Part model, mm, in its own coordinate system. Face numbers are marked on the shaded views. A direction names the side the tool comes from. Coordinates: 2 decimals unless noted, no trailing zeros. Write each loop counter-clockwise with the first axis right and the second up, starting at its lowest first coordinate (ties: lowest second). Pieces come first, ordered by that corner, then holes. Notation, with made-up numbers: M 69.5,-15.5 L 98.5,-15.5 A20 ccw 98.5,8.5 Z; hole C 53,40 d10. An arc over 180 degrees is marked long. Use a Markdown table: item, result. Add a question column.
Q1. Wall check: L1, parallel to Z at x = 0, y = 1.35; L2, parallel to Y at x = 0, z = -6.75; L3, parallel to Y at x = 6, z = -12. Give the ranges that are in metal, low to high. Write a range as from..to.
Q2. Slice it at B-B on y = -29. Write the cut outline in (x, z).
Q3. Tool access for the marked faces 1, 2, 3 and 4: list every direction of +Z, -Z, +X, -X, +Y, -Y with a clear straight run to the whole face (end or side of a thin tool).
Q4. Pin check, flat tips, straight feed: pin 1 Ø2.5 at (x, y) = (2, 18.5) entering from -Z; pin 2 Ø5 at (x, y) = (0, 50) entering from -Z; pin 3 Ø8 at (x, y) = (2.5, 32.5) entering from +Z. Stop position of each tip, or through.
Q5. Slice it at C-C on y = 7. Write the cut outline in (x, z), then the cut area to 3 significant figures.
Q6. Slice it at A-A on y = 50. Count the separate pieces of the cut face and the enclosed holes in it, then the cut area to 3 significant figures.
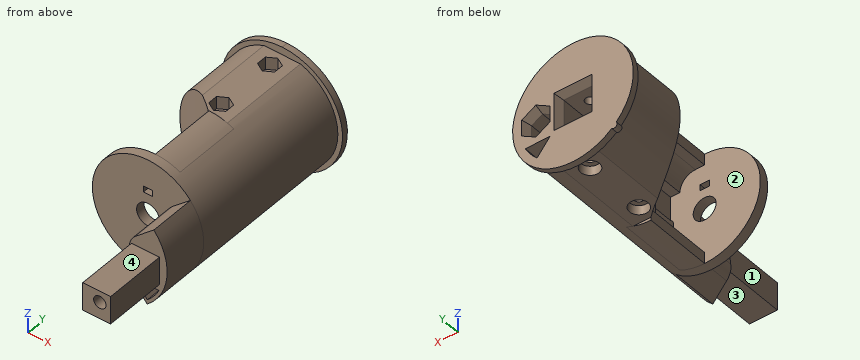
from build123d import *
from build123d.topology import SkipClean

# Parameters (mm, degrees)
SKETCH_1_R          = 18
EXTRUDE_1_DEPTH     = 55
SKETCH_2_R          = 19.5
EXTRUDE_2_DEPTH     = 2
SKETCH_3_W          = 10.25
SKETCH_3_H          = 10.25
CUT_EXTRUDE_1_DEPTH = 40
EXTRUDE_START       = 15
EXTRUDE_3_DEPTH     = 15
BOSS_EXTRUDE1_START = 20
SKETCH1_R           = 18
BOSS_EXTRUDE1_DEPTH = 20
BOSS_EXTRUDE2_START = 7
SKETCH3_R           = 18
BOSS_EXTRUDE2_DEPTH = 7
SKETCH4_W           = 10.2
SKETCH4_H           = 10.2
CUT_EXTRUDE2_DEPTH  = 27
CUT_EXTRUDE4_DEPTH  = 25
BOSS_EXTRUDE3_DEPTH = 3
SKETCH9_W           = 36
SKETCH9_H           = 22
CUT_EXTRUDE5_DEPTH  = 8
SKETCH10_R          = 3.7
SKETCH10_W          = 3
SKETCH10_H          = 2
CUT_EXTRUDE6_DEPTH  = 10
SKETCH11_R          = 2
CUT_EXTRUDE7_DEPTH  = 102
SKETCH15_R          = 18
CUT_EXTRUDE9_DEPTH  = 27
CUT_EXTRUDE11_DEPTH = 30
SKETCH18_R          = 1.5
CUT_EXTRUDE12_DEPTH = 71.437915926
SKETCH19_R          = 3
CUT_EXTRUDE13_DEPTH = 3
BOSS_EXTRUDE5_DEPTH = 22
CUT_EXTRUDE16_DEPTH = 4
CUT_EXTRUDE17_DEPTH = 25.4
CUT_EXTRUDE18_DEPTH = 71.437915926
FILLET2_R           = 5
SKETCH30_W          = 18.8
SKETCH30_H          = 10
CUT_EXTRUDE20_DEPTH = 3
CHAMFER1_SIZE       = 1
CHAMFER1_SIZE2      = 2.747477419
CHAMFER2_SIZE       = 1
CHAMFER2_SIZE2      = 2.747477419
BOSS_EXTRUDE7_START = 20
SKETCH37_W          = 9
SKETCH37_H          = 9
SKETCH37_R          = 2
BOSS_EXTRUDE7_DEPTH = 20
CUT_EXTRUDE22_DEPTH = 15
CUT_EXTRUDE23_DEPTH = 78.100583655
SKETCH40_W          = 4.363156696
SKETCH40_H          = 4.363156696
CUT_EXTRUDE24_DEPTH = 10
FILLET7_R           = 6
BOSS_EXTRUDE8_DEPTH = 2
CUT_EXTRUDE25_DEPTH = 12


with BuildPart() as part:
    # Эскиз1 → Бобышка-Вытянуть1 (new body)
    with BuildSketch(Plane(origin=(0, 0, 0), x_dir=(1, 0, 0), z_dir=(0, 1, 0))):
        with Locations(Location((0, 0, 0), (0, 0, 270))):
            Circle(SKETCH_1_R)
    extrude(amount=EXTRUDE_1_DEPTH)

    # Эскиз2 → Бобышка-Вытянуть2 (add)
    with BuildSketch(Plane(origin=(0, 55, 0), x_dir=(1, 0, 0), z_dir=(0, 1, 0))):
        with Locations(Location((0, 0, 0), (0, 0, 270))):
            Circle(SKETCH_2_R)
    extrude(amount=EXTRUDE_2_DEPTH)

    # Эскиз3 → Вырез-Вытянуть1 (cut)
    with BuildSketch(Plane(origin=(0, 57, 0), x_dir=(1, 0, 0), z_dir=(0, 1, 0))):
        Rectangle(SKETCH_3_W, SKETCH_3_H)
    extrude(amount=-CUT_EXTRUDE_1_DEPTH, mode=Mode.SUBTRACT)

    # Эскиз4 → Бобышка-Вытянуть3 (add)
    with SkipClean():  # the faces are left unmerged after this step: merging them gives an invalid solid
        with BuildSketch(Plane.XZ.offset(EXTRUDE_START)):
            with BuildLine():
                Line((5.142300877, -6.128355545), (11.570176974, -13.788799976))
                ThreePointArc((11.570176974, -13.788799976), (17.937391115, -1.5), (13.69961987, 11.675633406))
                Line((13.69961987, 11.675633406), (5.142300877, 4.38257561))
                Line((5.142300877, 4.38257561), (5.142300877, -6.128355545))
            make_face()
        extrude(amount=-EXTRUDE_3_DEPTH)

    # Sketch1 → Boss-Extrude1 (add)
    with BuildSketch(Plane.XZ.offset(15).offset(BOSS_EXTRUDE1_START)):
        with Locations(Location((0, 0, 0), (0, 0, 270))):
            Circle(SKETCH1_R)
    extrude(amount=-BOSS_EXTRUDE1_DEPTH)

    # Sketch3 → Boss-Extrude2 (add)
    with BuildSketch(Plane.XZ.offset(35).offset(BOSS_EXTRUDE2_START)):
        with Locations(Location((0, 0, 0), (0, 0, 270))):
            Circle(SKETCH3_R)
    extrude(amount=-BOSS_EXTRUDE2_DEPTH)

    # Sketch4 → Cut-Extrude2 (cut)
    with BuildSketch(Plane.XZ.offset(42)):
        Rectangle(SKETCH4_W, SKETCH4_H)
    extrude(amount=-CUT_EXTRUDE2_DEPTH, mode=Mode.SUBTRACT)

    # Sketch6 → Cut-Extrude4 (cut)
    with BuildSketch(Plane.XZ):
        with BuildLine():
            Line((0, 18), (0, -18))
            ThreePointArc((0, -18), (-18, 0), (0, 18))
        make_face()
    extrude(amount=-CUT_EXTRUDE4_DEPTH, mode=Mode.SUBTRACT)

    # Sketch8 → Boss-Extrude3 (add)
    with BuildSketch(Plane.XZ):
        with BuildLine():
            Line((0, -18), (0, 18))
            ThreePointArc((0, 18), (-18, 0), (0, -18))
        make_face()
    extrude(amount=-BOSS_EXTRUDE3_DEPTH)

    # Sketch9 → Cut-Extrude5 (cut)
    with BuildSketch(Plane.ZY):
        with Locations((0, 14)):
            Rectangle(SKETCH9_W, SKETCH9_H)
    extrude(amount=-CUT_EXTRUDE5_DEPTH, mode=Mode.SUBTRACT)

    # Sketch10 → Cut-Extrude6 (cut)
    with BuildSketch(Plane.XZ):
        with Locations(Location((0, 0, 0), (0, 0, 270))):
            Circle(SKETCH10_R)
        with Locations((0, 7.7)):
            Rectangle(SKETCH10_W, SKETCH10_H)
    extrude(amount=-CUT_EXTRUDE6_DEPTH, mode=Mode.SUBTRACT)

    # Sketch11 → Cut-Extrude7 (cut)
    with BuildSketch(Plane.XZ.offset(42)):
        with Locations(Location((12, 0, 0), (0, 0, 270))):
            Circle(SKETCH11_R)
    extrude(amount=-CUT_EXTRUDE7_DEPTH, mode=Mode.SUBTRACT)

    # Sketch15 → Cut-Extrude9 (cut)
    with BuildSketch(Plane.XZ.offset(42)):
        with Locations(Location((0, 0, 0), (0, 0, 310))):
            Circle(SKETCH15_R)
    extrude(amount=-CUT_EXTRUDE9_DEPTH, mode=Mode.SUBTRACT)

    # Sketch17 → Cut-Extrude11 (cut)
    with BuildSketch(Plane.XZ.offset(-25)):
        with BuildLine():
            Line((5.916079783, -17), (-5.916079783, -17))
            ThreePointArc((-5.916079783, -17), (0, -18), (5.916079783, -17))
        make_face()
        with BuildLine():
            Line((5.916079783, 17), (-5.916079783, 17))
            ThreePointArc((-5.916079783, 17), (0, 18), (5.916079783, 17))
        make_face()
    extrude(amount=-CUT_EXTRUDE11_DEPTH, mode=Mode.SUBTRACT)

    # Sketch18 → Cut-Extrude12 (cut, through all)
    with BuildSketch(Plane.XY.offset(-17)):
        with Locations(Location((0, 30, 0), (0, 0, 180))):
            Circle(SKETCH18_R)
        with Locations(Location((0, 50, 0), (0, 0, 180))):
            Circle(SKETCH18_R)
    extrude(amount=CUT_EXTRUDE12_DEPTH, mode=Mode.SUBTRACT)

    # Sketch19 → Cut-Extrude13 (cut)
    with BuildSketch(Plane.XY.offset(-17)):
        with Locations((0, 30)):
            Circle(SKETCH19_R)
        with Locations((0, 50)):
            Circle(SKETCH19_R)
    extrude(amount=CUT_EXTRUDE13_DEPTH, mode=Mode.SUBTRACT)

    # Sketch23 → Boss-Extrude5 (add)
    with BuildSketch(Plane(origin=(0, 3, 0), x_dir=(1, 0, 0), z_dir=(0, 1, 0))):
        with BuildLine():
            Line((0, -14.4), (8, -14.4))
            Line((8, -14.4), (8, -16.124515497))
            ThreePointArc((8, -16.124515497), (4.108449894, -17.524857759), (0, -18))
            Line((0, -18), (0, -14.4))
        make_face()
        with BuildLine():
            Line((0, 14.4), (8, 14.4))
            Line((8, 14.4), (8, 16.124515497))
            ThreePointArc((8, 16.124515497), (4.108449894, 17.524857759), (0, 18))
            Line((0, 18), (0, 14.4))
        make_face()
    extrude(amount=BOSS_EXTRUDE5_DEPTH)

    # Sketch25 → Cut-Extrude16 (cut)
    with BuildSketch(Plane.XY.offset(17)):
        Polygon((2.771281292, 28.4), (2.771281292, 31.6), (0, 33.2), (-2.771281292, 31.6), (-2.771281292, 28.4), (0, 26.8), align=None)
        Polygon((-2.782126929, 48.418933983), (-0.021820128, 46.800074394), (2.760306801, 48.381140412), (2.782126929, 51.581066017), (0.021820128, 53.199925606), (-2.760306801, 51.618859588), align=None)
    extrude(amount=-CUT_EXTRUDE16_DEPTH, mode=Mode.SUBTRACT)

    # Sketch26 → Cut-Extrude17 (cut)
    with BuildSketch(Plane(origin=(0, 57, 0), x_dir=(1, 0, 0), z_dir=(0, 1, 0))):
        Polygon((8.449295844, -2.05), (12, -4.1), (15.550704156, -2.05), (15.550704156, 2.05), (12, 4.1), (8.449295844, 2.05), align=None)
    extrude(amount=-CUT_EXTRUDE17_DEPTH, mode=Mode.SUBTRACT)

    # Sketch27 → Cut-Extrude18 (cut, through all)
    with BuildSketch(Plane.XY.offset(17)):
        with BuildLine():
            Line((-20, 36.547005384), (-20, 25))
            Line((-20, 25), (0, 25))
            ThreePointArc((0, 25), (-9.324199199, 31.944024015), (-20, 36.547005384))
        make_face()
    extrude(amount=-CUT_EXTRUDE18_DEPTH, mode=Mode.SUBTRACT)

    # Fillet2
    fillet2_edges = [part.edges().sort_by_distance(p)[0] for p in [
        (8, 14, -14.4),
        (8, 14, 14.4),
    ]]
    fillet(fillet2_edges, radius=FILLET2_R)

    # Sketch30 → Cut-Extrude20 (cut)
    with BuildSketch(Plane.ZY.offset(-8)):
        with Locations((0, 8)):
            Rectangle(SKETCH30_W, SKETCH30_H)
    extrude(amount=-CUT_EXTRUDE20_DEPTH, mode=Mode.SUBTRACT)

    # Chamfer1
    chamfer1_edges = [part.edges().sort_by_distance(p)[0] for p in [
        (5.125, 57, 0),
        (0, 57, -5.125),
        (-5.125, 57, 0),
        (0, 57, 5.125),
    ]]
    chamfer1_side = [part.faces().sort_by_distance(p)[0] for p in [
        (0, 57, -18.948456711),
    ]]
    chamfer(chamfer1_edges, length=CHAMFER1_SIZE, length2=CHAMFER1_SIZE2, reference=chamfer1_side[0])

    # Chamfer2
    chamfer2_edges = [part.edges().sort_by_distance(p)[0] for p in [
        (8.449295844, 57, 0),
        (10.224647922, 57, 3.075),
        (13.775352078, 57, 3.075),
        (15.550704156, 57, 0),
        (13.775352078, 57, -3.075),
        (10.224647922, 57, -3.075),
    ]]
    chamfer2_side = [part.faces().sort_by_distance(p)[0] for p in [
        (6.676543289, 57, 0),
    ]]
    chamfer(chamfer2_edges, length=CHAMFER2_SIZE, length2=CHAMFER2_SIZE2, reference=chamfer2_side[0])

    # Sketch37 → Boss-Extrude7 (add)
    with BuildSketch(Plane.XZ.offset(15).offset(BOSS_EXTRUDE7_START)):
        with Locations((10.978822628, -0.872889968)):
            Rectangle(SKETCH37_W, SKETCH37_H)
        with Locations(Location((12, 0, 0), (0, 0, 270))):
            Circle(SKETCH37_R, mode=Mode.SUBTRACT)
    extrude(amount=-BOSS_EXTRUDE7_DEPTH)

    # Sketch38 → Cut-Extrude22 (cut)
    with BuildSketch(Plane.XZ.offset(15)):
        with BuildLine():
            Line((5.142300877, -6.128355545), (5.142300877, 4.38257561))
            ThreePointArc((5.142300877, 4.38257561), (5.978822628, -0.872889968), (5.142300877, -6.128355545))
        make_face()
    extrude(amount=-CUT_EXTRUDE22_DEPTH, mode=Mode.SUBTRACT)

    # Sketch39 → Cut-Extrude23 (cut, through all)
    with BuildSketch(Plane.XZ.offset(15)):
        with BuildLine():
            Line((7.420733648, -7.372889968), (15.420733648, -7.372889968))
            ThreePointArc((15.420733648, -7.372889968), (13.728515389, -10.030415688), (11.598853111, -12.352178848))
            Line((11.598853111, -12.352178848), (7.420733648, -7.372889968))
        make_face()
    extrude(amount=-CUT_EXTRUDE23_DEPTH, mode=Mode.SUBTRACT)

    # Sketch40 → Cut-Extrude24 (cut)
    with BuildSketch(Plane(origin=(0, 3, 0), x_dir=(1, 0, 0), z_dir=(0, 1, 0))):
        with Locations((9.602311996, 9.554468316)):
            Rectangle(SKETCH40_W, SKETCH40_H)
    extrude(amount=CUT_EXTRUDE24_DEPTH, mode=Mode.SUBTRACT)

    # Fillet7
    fillet7_edges = [part.edges().sort_by_distance(p)[0] for p in [
        (5.142300877, -7.5, 4.38257561),
        (5.142300877, -7.5, -6.128355545),
    ]]
    fillet(fillet7_edges, radius=FILLET7_R)

    # Sketch41 → Boss-Extrude8 (add)
    with BuildSketch(Plane(origin=(0, 57, 0), x_dir=(1, 0, 0), z_dir=(0, 1, 0))):
        with BuildLine():
            Line((-13.998504433, 13.575414308), (-12.534358389, 14.937866641))
            ThreePointArc((-12.534358389, 14.937866641), (-13.947657578, 14.988713497), (-13.998504433, 13.575414308))
        make_face()
    extrude(amount=-BOSS_EXTRUDE8_DEPTH)

    # Sketch42 → Cut-Extrude25 (cut)
    with BuildSketch(Plane.XZ.offset(-13)):
        Polygon((8, -8.063232724), (7.420733648, -11.736046664), (11.081856822, -11.736046664), align=None)
    extrude(amount=-CUT_EXTRUDE25_DEPTH, mode=Mode.SUBTRACT)


solid = part.part
Recorded:
| question | item | result |
|---|---|---|
| 1 | L1 | -18..-3.7, 3.7..6.7, 8.7..18 |
| 1 | L2 | 0..3, 25..28.5, 31.5..48.5, 51.5..57 |
| 1 | L3 | 0..3, 25..57 |
| 2 | outline | M 6.48,-5.37 L 15.48,-5.37 L 15.48,3.63 L 6.48,3.63 Z; hole C 12,0 d4 |
| 3 | face 1 | +Z, -Z, -X, -Y |
| 3 | face 2 | -X |
| 3 | face 3 | -Z, +X, -X, -Y |
| 3 | face 4 | +Z, +X, -X, -Y |
| 4 | pin 1 | z = -17.98 |
| 4 | pin 2 | z = -14 |
| 4 | pin 3 | z = 17 |
| 5 | outline | M 0,-18 A18 ccw 0,18 L 0,14.4 L 3,14.4 A5 cw 8,9.4 L 11,9.4 L 11,1.73 A2 cw long 11,-1.73 L 11,-7.37 L 15.42,-7.37 A18 cw 11.6,-12.35 L 11.08,-11.74 L 7.42,-11.74 A5 cw 3,-14.4 L 0,-14.4 Z |
| 5 | area | 202 mm² |
| 6 | separate pieces | 2 |
| 6 | enclosed holes | 2 |
| 6 | area | 742 mm² |
